Build history of the part. All positions in model axes, mm. Face numbers are marked on the shaded views. Give positions to 0.01 mm unless a question says otherwise; leave off trailing zeros. Loops run counter-clockwise (first coordinate to the right, second up) from the corner with the lowest first, then second, coordinate; pieces in that order, holes last.
1) Flat gauge pins, fed straight in: P1, Ø2, axis at x = -56.5, z = 10.5, coming from the +Y side; P2, Ø1.5, axis at x = -87.5, z = 4.5, coming from the +Y side; P3, Ø12, axis at x = -86, y = 3.5, coming from the +Z side. Where does each tip first touch, or does it go through?
2) Wall check: line 1 (Y direction, x = 6, z = 4); line 2 (X direction, y = 4, z = 6.5); line 3 (X direction, y = -2.25, z = 11.25). Give the ranges that are in metal, low to high.
3) Band-saw the part on B-B on x = -36. List the corners of the cut face in (y, z), then the cut area to 3 significant figures.
4) Two-plate mould, pull along Y, no slides. Class the marked faces 1, 2 and 3: +Y half, -Y half, draft (parallel to the pull), parting line (faces both ways), or undercut.
5) Band-saw the part on A-A on z = 6. List the corners of the cut face in (x, y).
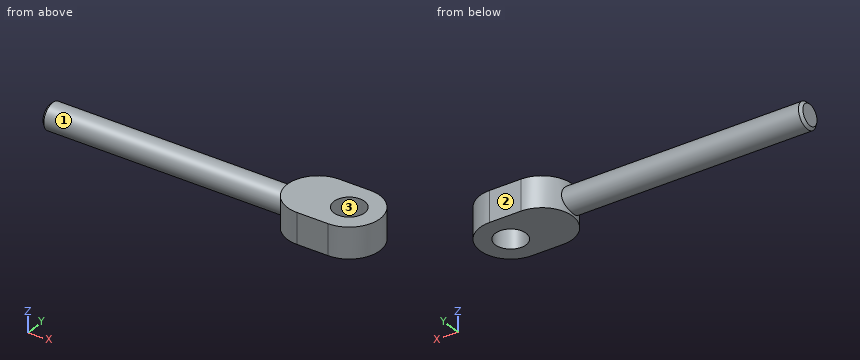
```python
from build123d import *

# Parameters (mm, degrees)
SCHIZZO1_R                        = 6
ESTRUSIONE_ESTRUSIONE1_DEPTH      = 12
ESTRUSIONE_ESTRUSIONE2_REACH      = 130.129
ESTRUSIONE_ESTRUSIONE2_END_RADIUS = 12
SCHIZZO2_R                        = 5
SMUSSO1_SIZE                      = 1


with BuildPart() as part:
    # Schizzo1 → Estrusione-Estrusione1 (new body)
    with BuildSketch(Plane.XY):
        with BuildLine():
            Line((-6, 12), (6, 12))
            ThreePointArc((6, 12), (18, 0), (6, -12))
            Line((6, -12), (-6, -12))
            ThreePointArc((-6, -12), (-18, 0), (-6, 12))
        make_face()
        with Locations((6, 0)):
            Circle(SCHIZZO1_R, mode=Mode.SUBTRACT)
    extrude(amount=ESTRUSIONE_ESTRUSIONE1_DEPTH)

    # Estrusione-Estrusione2: up to this cylinder (the profile starts outside it)
    estrusione_estrusione2_end = Plane(origin=(-6, 0, 6), z_dir=(0, 0, -1)) * Cylinder(ESTRUSIONE_ESTRUSIONE2_END_RADIUS, 285.258, mode=Mode.PRIVATE)
    # Schizzo2 → Estrusione-Estrusione2 (add, up to the surface)
    with BuildSketch(Plane(origin=(-109, 0, 0), x_dir=(0, 0, -1), z_dir=(1, 0, 0)), mode=Mode.PRIVATE) as estrusione_estrusione2_sk1:
        with Locations(Location((-6, 0, 0), (0, 0, 180))):
            Circle(SCHIZZO2_R)
    estrusione_estrusione2_tool1 = extrude(estrusione_estrusione2_sk1.sketch, amount=ESTRUSIONE_ESTRUSIONE2_REACH, mode=Mode.PRIVATE) - estrusione_estrusione2_end
    add(estrusione_estrusione2_tool1.solids().sort_by_distance((-109, 0, 6))[0])

    # Smusso1
    smusso1_edges = [part.edges().sort_by_distance(p)[0] for p in [
        (-109, 0, 1),
    ]]
    chamfer(smusso1_edges, length=SMUSSO1_SIZE)


solid = part.part
```
Findings below:
1. P1: stops at y = 3.57
1. P2: stops at y = 4.94
1. P3: stops at z = 11
2. line 1: y = -12 to -6, 6 to 12
2. line 2: x = -108.97 to 1.53, 10.47 to 17.31
2. line 3: x = -17.79 to 0.44, 11.56 to 17.79
3. outline: circle Ø10 at (0, 6)
3. area: 78.5 mm2
4. face 1: parting line
4. face 2: +Y half
4. face 3: undercut
5. outline: (-109, -4) - (-108, -5) - (-16.91, -5) arc R12 ccw to (-6, -12) - (6, -12) arc R12 ccw to (6, 12) - (-6, 12) arc R12 ccw to (-16.91, 5) - (-108, 5) - (-109, 4) - close; hole circle Ø12 at (6, 0)
